Check sheet for the modelled part. Datum: model origin and axes. Units: mm. Give positions to 0.01 mm unless a question says otherwise; leave off trailing zeros. Order: outer loops, then holes, each group sorted by start corner. A loop starts at its lowest first (then second) coordinate and runs counter-clockwise, first axis right, second up.
```python
from build123d import *

# Parameters (mm, degrees)
SKETCH1_R           = 57
SKETCH1_R_2         = 44.5
BOSS_EXTRUDE1_DEPTH = 3
CUT_EXTRUDE1_REACH  = 82.666
SKETCH3_W           = 8
SKETCH3_H           = 3
CIRPATTERN1_COUNT   = 14


with BuildPart() as part:
    # Sketch1 → Boss-Extrude1 (new body)
    with BuildSketch(Plane.XY):
        Circle(SKETCH1_R)
        Circle(SKETCH1_R_2, mode=Mode.SUBTRACT)
    extrude(amount=BOSS_EXTRUDE1_DEPTH)

    # Sketch3 → Cut-Extrude1 (cut, up to next)
    with BuildSketch(Plane.XY.offset(3), mode=Mode.PRIVATE) as cut_extrude1_sk1:
        with Locations((0, 45.819860108)):
            Rectangle(SKETCH3_W, SKETCH3_H)
    cut_extrude1_tool1 = extrude(cut_extrude1_sk1.sketch, amount=-CUT_EXTRUDE1_REACH, mode=Mode.PRIVATE) & part.part
    cut_extrude1 = cut_extrude1_tool1.solids().sort_by_distance((0, 45.81986, 3))[0]
    add(cut_extrude1, mode=Mode.SUBTRACT)

    # CirPattern1: Cut-Extrude1 ×14 about axis
    cirpattern1_axis = Axis((0, 0, 0), (0, 0, 1))
    for i in range(1, CIRPATTERN1_COUNT):
        add(cut_extrude1.rotate(cirpattern1_axis, i * 360 / CIRPATTERN1_COUNT), mode=Mode.SUBTRACT)


solid = part.part
```
Q1. Go/stop test with flat-tipped pins: P1, Ø1.5, axis at y = -45.5, z = 1, coming from the -X side; P2, Ø1.5, axis at x = 28.5, z = 2, coming from the -Y side; P3, Ø0.9, axis at x = 1.5, z = 1, coming from the -Y side; P4, Ø5, axis at x = 31.5, y = -27.5, coming from the -Z side. Record where each tip stops, or that it passes through.
Q2. Material ranges on line 1 (Y direction, x = 0, z = 1.9); line 2 (Y direction, x = -45, z = 0.3); line 3 (Y direction, x = -23, z = 2.1), recorded low to high.
Q3. Sectioned sample at A-A, the plane y = 0. Record the cut outline in (x, z), plus the area to 3 significant figures.
Q4. Sectioned sample at B-B, the plane x = 0. Record the cut outline in (y, z), plus the area to 3 significant figures.
Filled in:
1. P1: stops at x = -35.3
1. P2: stops at y = -49.79
1. P3: stops at y = -56.99
1. P4: passes through
2. line 1: y = -57 to -47.32, 47.32 to 57
2. line 2: y = -34.99 to -14.37, -6.17 to 6.17, 14.37 to 34.99
2. line 3: y = -52.15 to -41.44, -38.54 to -38.1, 38.1 to 38.54, 41.44 to 52.15
3. outline: (-57, 0) - (-44.5, 0) - (-44.5, 3) - (-57, 3) - close; (44.5, 0) - (57, 0) - (57, 3) - (44.5, 3) - close
3. area: 75.0 mm2
4. outline: (-57, 0) - (-47.32, 0) - (-47.32, 3) - (-57, 3) - close; (47.32, 0) - (57, 0) - (57, 3) - (47.32, 3) - close
4. area: 58.1 mm2
